from build123d import *

# Parameters (mm, degrees)
CROQUIS1_R                   = 30.165
SALIENTE_EXTRUIR1_DEPTH      = 2
SALIENTE_EXTRUIR1_DEPTH_BACK = 2
CROQUIS3_R                   = 26.25
CROQUIS3_R_2                 = 23.25
SALIENTE_EXTRUIR2_DEPTH      = 5


with BuildPart() as part:
    # Croquis1 → Saliente-Extruir1 (new body, two sides)
    with BuildSketch(Plane.XY) as saliente_extruir1_sk:
        Circle(CROQUIS1_R)
    extrude(amount=SALIENTE_EXTRUIR1_DEPTH)
    extrude(saliente_extruir1_sk.sketch, amount=-SALIENTE_EXTRUIR1_DEPTH_BACK)

    # Croquis3 → Saliente-Extruir2 (add)
    with BuildSketch(Plane.XY.offset(2)):
        Circle(CROQUIS3_R)
        Circle(CROQUIS3_R_2, mode=Mode.SUBTRACT)
    extrude(amount=SALIENTE_EXTRUIR2_DEPTH)


solid = part.part
Design review of the part built by this model. Coordinates are the model's own, in mm. A direction names the side the tool comes from. Give positions to 0.01 mm unless a question says otherwise; leave off trailing zeros. Loops run counter-clockwise (first coordinate to the right, second up) from the corner with the lowest first, then second, coordinate; pieces in that order, holes last. Notation, with made-up numbers: (57.25, 80.25) - (112.25, 80.25) arc R24 cw to (112.25, 116.25) - close; hole circle Ø4 at (-24.75, -12). An arc over 180 degrees is marked (long way). Use CSV: the item, a comma, the result in double quotes. Start each with the question number.
1. Insertion check: P1, Ø1, axis at x = 15, z = -0.5, coming from the +Y side; P2, Ø1.5, axis at x = -2.5, z = 6, coming from the +Y side; P3, Ø12, axis at x = 9.5, y = 7.5, coming from the +Z side. Each pin has a flat end and moves straight along its axis. Give the tip position at first contact, or say it passes through.
2. Machinability: for faces 4 (the cylindrical face through (22.176, 6.984, 4.465)), 5 (the flat face through (0, 0, -2)), which of the approach directions +Z, -Z, +X, -X, +Y, -Y give a long, thin tool a straight path to every point of the face, cutting with its end or side? Answer none if there is none.
3. Wall thickness on L1, parallel to Y at x = 0, z = 5.2; L2, parallel to Z at x = 5, y = 11; L3, parallel to Y at x = 0, z = 1.5 (3 decimals): over which ranges is each line inside the solid? List them lowest first.
4. Add section A-A (y = 0). State the section outline as (x, z) points (3 decimals).
5. Add section C-C (z = 2.75). State the section outline as (x, y) points, plus the area to 3 significant figures.
6. Draft analysis for pull direction X (two halves, no side actions). For faces 1 (the cylindrical face through (25, 8, 4)), 2 (the flat face through (-15.7, -17.4, 7)), 3 (the flat face through (0, 0, 2)), state which applies: released by +X, released by -X, zero draft, split by the parting line, or undercut.
Results found:
1,P1,"stops at y = 26.45"
1,P2,"stops at y = 26.19"
1,P3,"stops at z = 2"
2,face 4,"+Z"
2,face 5,"-Z, +X, -X, +Y, -Y"
3,L1,"y = -26.25 to -23.25, 23.25 to 26.25"
3,L2,"z = -2 to 2"
3,L3,"y = -30.165 to 30.165"
4,outline,"(-30.165, -2) - (30.165, -2) - (30.165, 2) - (26.25, 2) - (26.25, 7) - (23.25, 7) - (23.25, 2) - (-23.25, 2) - (-23.25, 7) - (-26.25, 7) - (-26.25, 2) - (-30.165, 2) - close"
5,outline,"circle Ø52.5 at (0, 0); hole circle Ø46.5 at (0, 0)"
5,area,"467 mm²"
6,face 1,"split by the parting line"
6,face 2,"zero draft"
6,face 3,"undercut"
